Design review of the part shown in the three views and the two pictorial views. Dimensions are in mm from the part's minimum x, y and z. Give positions to 0.01 mm unless a question says otherwise; leave off trailing zeros. Order: outer loops, then holes, each group sorted by start corner. A loop starts at its lowest first (then second) coordinate and runs counter-clockwise, first axis right, second up. Notation, with made-up numbers: M 73.5,17.5 L 103.5,17.5 A13 ccw 103.5,41.5 Z; hole C 45.25,-2.5 d1. An arc over 180 degrees is marked long. Answer as a JSON object with one key per item and string values.
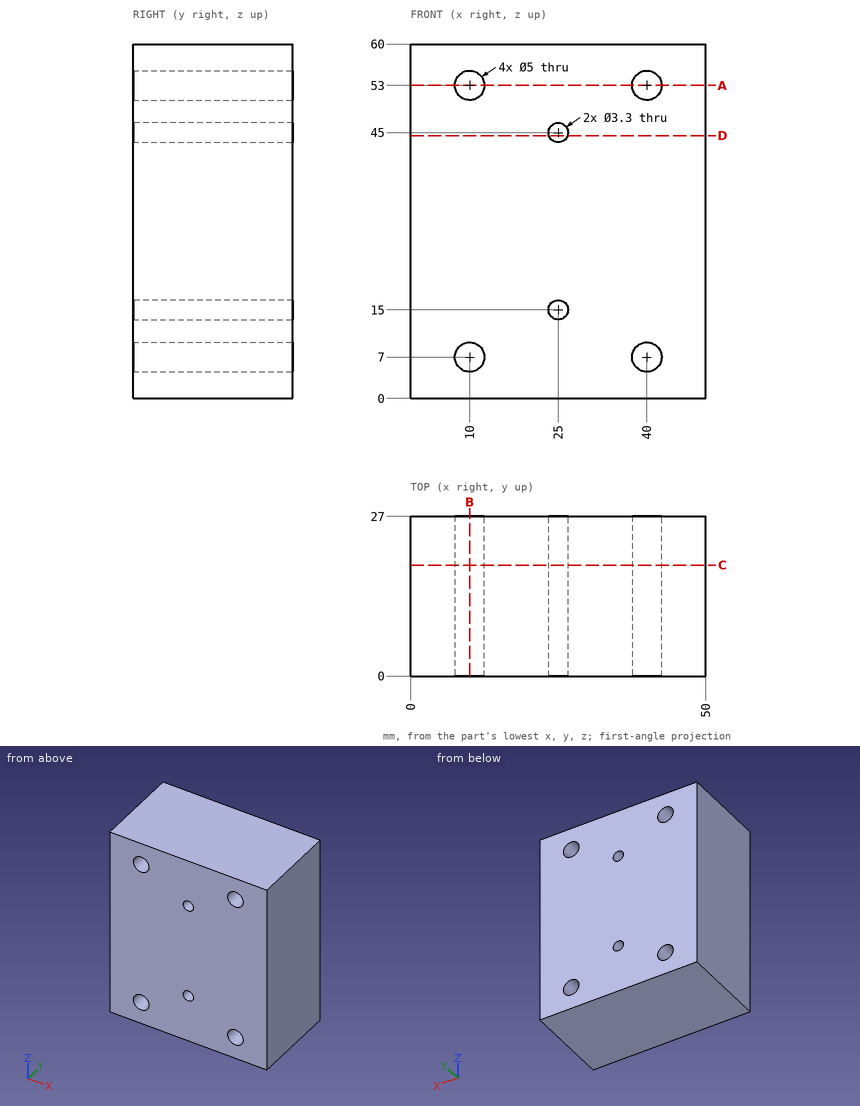
(1) Insertion check: pin 1 (4.5 mm diameter, centred on x = 40, z = 7, fed in from +Y). The pin has a flat end and moves straight along its axis. Give the tip position at first contact, or say it passes through.
Checked values:
{"pin 1": "passes through"}
(2) We need section C-C (y = 18.75). Write out the cut boundary in (x, z), plus the area to 3 significant figures.
Checked values:
{"outline": "M 0,0 L 50,0 L 50,60 L 0,60 Z; hole C 10,7 d5; hole C 10,53 d5; hole C 25,15 d3.3; hole C 25,45 d3.3; hole C 40,7 d5; hole C 40,53 d5", "area": "2,900 mm^2"}
(3) We need section A-A (z = 53). Write out the cut boundary in (x, y), plus the area to 3 significant figures.
Checked values:
{"outline": "M 0,0 L 7.5,0 L 7.5,27 L 0,27 Z; M 12.5,0 L 37.5,0 L 37.5,27 L 12.5,27 Z; M 42.5,0 L 50,0 L 50,27 L 42.5,27 Z", "area": "1,080 mm^2"}
(4) We need section D-D (z = 44.5). Write out the cut boundary in (x, y).
Checked values:
{"outline": "M 0,0 L 23.43,0 L 23.43,27 L 0,27 Z; M 26.57,0 L 50,0 L 50,27 L 26.57,27 Z"}
(5) We need section B-B (x = 10). Write out the cut boundary in (y, z), plus the area to 3 significant figures.
Checked values:
{"outline": "M 0,0 L 27,0 L 27,4.5 L 0,4.5 Z; M 0,9.5 L 27,9.5 L 27,50.5 L 0,50.5 Z; M 0,55.5 L 27,55.5 L 27,60 L 0,60 Z", "area": "1,350 mm^2"}
(6) To check wall thickness, follow L1, parallel to Z at x = 40, y = 11.75; L2, parallel to X at y = 13.25, z = 51.5; L3, parallel to Z at x = 10.5, y = 5.25. State the ranges of each line that lie inside material, in increasing order. Write a range as from..to.
Checked values:
{"L1": "z = 0..4.5, 9.5..50.5, 55.5..60", "L2": "x = 0..8, 12..38, 42..50", "L3": "z = 0..4.55, 9.45..50.55, 55.45..60"}
